```python
from build123d import *

# Parameters (mm, degrees)
EXTRUDE_RAIL_PROFILE_DEPTH        = 300
INITIAL_MOUNTING_HOLE_D           = 3.5
INITIAL_MOUNTING_HOLE_CBORE_D     = 6
INITIAL_MOUNTING_HOLE_CBORE_DEPTH = 4
FILL_START                        = -2.2
FILL_PATTERN_OUTLINE_R            = 3
FILL_PATTERN_DEPTH                = 4
FILL_START_2                      = -4.7
FILL_PATTERN_2_OUTLINE_R          = 1.75
FILL_PATTERN_2_DEPTH              = 2.5


# Read off the part's stored shape, not the designer's step: Fill Pattern
with BuildPart() as part:
    # Rail Profile Sketch → Extrude Rail Profile (new body)
    with BuildSketch(Plane.XY):
        with BuildLine():
            Line((-4.3, -4.7), (4.3, -4.7))
            Line((4.3, -4.7), (4.5, -4.5))
            Line((4.5, -4.5), (4.5, -0.994987437))
            ThreePointArc((4.5, -0.994987437), (3.948817336, -0.758921035), (3.631754163, -0.25))
            Line((3.631754163, -0.25), (3.131754163, -0.25))
            Line((3.131754163, -0.25), (3.131754163, 0.25))
            Line((3.131754163, 0.25), (3.631754163, 0.25))
            ThreePointArc((3.631754163, 0.25), (3.948817336, 0.758921035), (4.5, 0.994987437))
            Line((4.5, 0.994987437), (4.5, 1.6))
            Line((4.5, 1.6), (4.3, 1.8))
            Line((4.3, 1.8), (-4.3, 1.8))
            Line((-4.3, 1.8), (-4.5, 1.6))
            Line((-4.5, 1.6), (-4.5, 0.994987437))
            ThreePointArc((-4.5, 0.994987437), (-3.948817336, 0.758921035), (-3.631754163, 0.25))
            Line((-3.631754163, 0.25), (-3.131754163, 0.25))
            Line((-3.131754163, 0.25), (-3.131754163, -0.25))
            Line((-3.131754163, -0.25), (-3.631754163, -0.25))
            ThreePointArc((-3.631754163, -0.25), (-3.948817336, -0.758921035), (-4.5, -0.994987437))
            Line((-4.5, -0.994987437), (-4.5, -4.5))
            Line((-4.5, -4.5), (-4.3, -4.7))
        make_face()
    extrude(amount=EXTRUDE_RAIL_PROFILE_DEPTH)

    # Initial Mounting Hole (through all)
    with Locations(Plane(origin=(0, 1.8, 0), x_dir=(1, 0, 0), z_dir=(0, 1, 0))):
        with Locations((0, -140)):
            CounterBoreHole(INITIAL_MOUNTING_HOLE_D / 2, INITIAL_MOUNTING_HOLE_CBORE_D / 2, INITIAL_MOUNTING_HOLE_CBORE_DEPTH)

    # Fill Pattern outline → Fill Pattern (cut)
    with BuildSketch(Plane(origin=(0, 0, 0), x_dir=(1, 0, 0), z_dir=(0, 1, 0)).offset(FILL_START)):
        with Locations((0, -120)):
            Circle(FILL_PATTERN_OUTLINE_R)
        with Locations((0, -160)):
            Circle(FILL_PATTERN_OUTLINE_R)
        with Locations((0, -100)):
            Circle(FILL_PATTERN_OUTLINE_R)
        with Locations((0, -180)):
            Circle(FILL_PATTERN_OUTLINE_R)
        with Locations((0, -80)):
            Circle(FILL_PATTERN_OUTLINE_R)
        with Locations((0, -200)):
            Circle(FILL_PATTERN_OUTLINE_R)
        with Locations((0, -60)):
            Circle(FILL_PATTERN_OUTLINE_R)
        with Locations((0, -220)):
            Circle(FILL_PATTERN_OUTLINE_R)
        with Locations((0, -40)):
            Circle(FILL_PATTERN_OUTLINE_R)
        with Locations((0, -240)):
            Circle(FILL_PATTERN_OUTLINE_R)
        with Locations((0, -20)):
            Circle(FILL_PATTERN_OUTLINE_R)
        with Locations((0, -260)):
            Circle(FILL_PATTERN_OUTLINE_R)
        with Locations((0, -280)):
            Circle(FILL_PATTERN_OUTLINE_R)
    extrude(amount=FILL_PATTERN_DEPTH, mode=Mode.SUBTRACT)

    # Fill Pattern 2 outline → Fill Pattern 2 (cut)
    with BuildSketch(Plane(origin=(0, 0, 0), x_dir=(1, 0, 0), z_dir=(0, 1, 0)).offset(FILL_START_2)):
        with Locations((0, -120)):
            Circle(FILL_PATTERN_2_OUTLINE_R)
        with Locations((0, -160)):
            Circle(FILL_PATTERN_2_OUTLINE_R)
        with Locations((0, -100)):
            Circle(FILL_PATTERN_2_OUTLINE_R)
        with Locations((0, -180)):
            Circle(FILL_PATTERN_2_OUTLINE_R)
        with Locations((0, -80)):
            Circle(FILL_PATTERN_2_OUTLINE_R)
        with Locations((0, -200)):
            Circle(FILL_PATTERN_2_OUTLINE_R)
        with Locations((0, -60)):
            Circle(FILL_PATTERN_2_OUTLINE_R)
        with Locations((0, -220)):
            Circle(FILL_PATTERN_2_OUTLINE_R)
        with Locations((0, -40)):
            Circle(FILL_PATTERN_2_OUTLINE_R)
        with Locations((0, -240)):
            Circle(FILL_PATTERN_2_OUTLINE_R)
        with Locations((0, -20)):
            Circle(FILL_PATTERN_2_OUTLINE_R)
        with Locations((0, -260)):
            Circle(FILL_PATTERN_2_OUTLINE_R)
        with Locations((0, -280)):
            Circle(FILL_PATTERN_2_OUTLINE_R)
    extrude(amount=FILL_PATTERN_2_DEPTH, mode=Mode.SUBTRACT)


solid = part.part
```
Design review of the part built by this model. Coordinates are the model's own, in mm. A direction names the side the tool comes from. Round coordinates to 2 decimals unless told otherwise and drop trailing zeros. Write each loop counter-clockwise with the first axis right and the second up, starting at its lowest first coordinate (ties: lowest second). Pieces come first, ordered by that corner, then holes.
Item 1: For faces 3 (the cylindrical face through (0, 0, 217)), 4 (the flat face through (0, -4.7, 148)), list the 3-axis set-ups (+Z, -Z, +X, -X, +Y, -Y) from which the entire face can be reached by the end or side of a thin tool; tool diameter is ignored.
Item 2: Clearance check with flat-ended pins moving along their axes: pin 1 Ø3 at (x, z) = (0.5, 201) entering from +Y; pin 2 Ø0.6 at (y, z) = (0, 143.5) entering from +X. State where each tip first meets the part, or that it passes through.
Item 3: We need section B-B on z = 269.5. Write out the cut boundary in (x, y), and give its area (3 significant figures).
Item 4: We need section A-A on y = -3.5. State how many separate pieces and enclosed holes the cut face has, and give its area (3 significant figures).
Item 5: The part is to be moulded in two halves that separate along Z. For faces 1 (the cylindrical face through (0, 0, 237)), 2 (the flat face through (0, 1.8, 148)), say which applies: +Z half, -Z half, draft (parallel to the pull), parting line (faces both ways), or undercut.
Item 6: For probe 1 along X at (y, z) = (-3.4, 280); probe 2 along Y at (x, z) = (3.5, 155); probe 3 along Y at (x, z) = (-2.5, 220), list the stretches that pass through material, from the lowest coordinate up.
Returned:
1. face 3: +Y
1. face 4: +Z, -Z, +X, -X, -Y
2. pin 1: stops at y = -2.2
2. pin 2: stops at x = 3.65
3. outline: (-4.5, -4.5) - (-4.3, -4.7) - (4.3, -4.7) - (4.5, -4.5) - (4.5, -0.99) arc R1 cw to (3.63, -0.25) - (3.13, -0.25) - (3.13, 0.25) - (3.63, 0.25) arc R1 cw to (4.5, 0.99) - (4.5, 1.6) - (4.3, 1.8) - (-4.3, 1.8) - (-4.5, 1.6) - (-4.5, 0.99) arc R1 cw to (-3.63, 0.25) - (-3.13, 0.25) - (-3.13, -0.25) - (-3.63, -0.25) arc R1 cw to (-4.5, -0.99) - close
3. area: 55.2 mm2
4. separate pieces: 1
4. enclosed holes: 14
4. area: 2,570 mm2
5. face 1: undercut
5. face 2: draft
6. probe 1: x = -4.5 to -1.75, 1.75 to 4.5
6. probe 2: y = -4.7 to -0.25, 0.25 to 1.8
6. probe 3: y = -4.7 to -2.2
